Read the model definition and answer for the solid it produces. Units are mm, in the model's axes. Coordinates: 2 decimals unless noted, no trailing zeros. Order: outer loops, then holes, each group sorted by start corner. A loop starts at its lowest first (then second) coordinate and runs counter-clockwise, first axis right, second up. Notation, with made-up numbers: M 26,38 L 40,38 A24 cw 40,54 Z; hole C -3,12 d9. An arc over 180 degrees is marked long. Use a Markdown table: item, result. Add a question column.
1) Find the intervals of material crossed by probe 1 along Y at (x, z) = (-12.5, 24) (3 decimals); probe 2 along X at (y, z) = (-266.5, 21) (3 decimals); probe 3 along Y at (x, z) = (30, 12.5) (3 decimals), in increasing order. Write a range as [from, to].
2) Find section B-B on x = 30. Write down the section's boundary in (y, z) (3 decimals), plus the area to 3 significant figures.
3) Find section A-A on z = 12.75. Write down the section's boundary in (x, y) (3 decimals), plus the area to 3 significant figures.
4) This flat-tipped pin is pushed along its axis until it touches: pin 1 Ø3 at (x, z) = (-5, 15) entering from +Y (3 decimals). Where does it stop, or does it pass through?
from build123d import *

# Parameters (mm, degrees)
SKETCH1_W           = 76.2
SKETCH1_H           = 641.35
BOSS_EXTRUDE1_DEPTH = 25.4
CUT_EXTRUDE1_DEPTH  = 25.4
CUT_EXTRUDE2_DEPTH  = 25.4


with BuildPart() as part:
    # Sketch1 → Boss-Extrude1 (new body)
    with BuildSketch(Plane.XY):
        Rectangle(SKETCH1_W, SKETCH1_H)
    extrude(amount=BOSS_EXTRUDE1_DEPTH)

    # Sketch2 → Cut-Extrude1 (cut)
    with BuildSketch(Plane.XY.offset(25.4)):
        Polygon((-38.1, -320.675), (38.1, -244.475), (38.1, -320.675), align=None)
    extrude(amount=-CUT_EXTRUDE1_DEPTH, mode=Mode.SUBTRACT)

    # Sketch3 → Cut-Extrude2 (cut)
    with BuildSketch(Plane.XY.offset(25.4)):
        Polygon((-38.1, 320.675), (38.1, 244.475), (38.1, 320.675), align=None)
    extrude(amount=-CUT_EXTRUDE2_DEPTH, mode=Mode.SUBTRACT)


solid = part.part
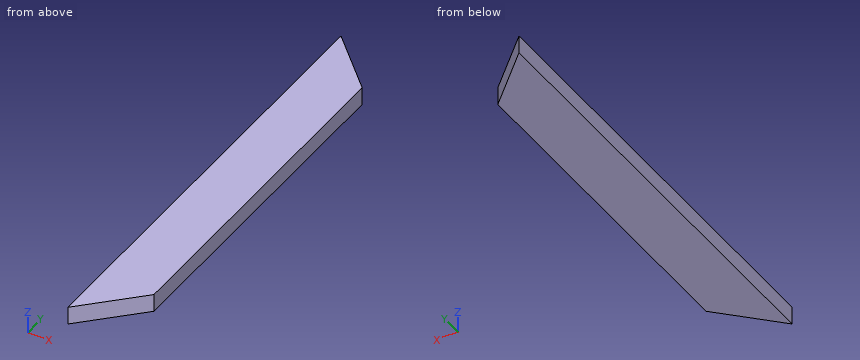
Check result:
| question | item | result |
|---|---|---|
| 1 | probe 1 | y = [-295.075, 295.075] |
| 1 | probe 2 | x = [-38.1, 16.075] |
| 1 | probe 3 | y = [-252.575, 252.575] |
| 2 | outline | M -252.575,0 L 252.575,0 L 252.575,25.4 L -252.575,25.4 Z |
| 2 | area | 12,800 mm2 |
| 3 | outline | M -38.1,-320.675 L 38.1,-244.475 L 38.1,244.475 L -38.1,320.675 Z |
| 3 | area | 43,100 mm2 |
| 4 | pin 1 | stops at y = 289.075 |
